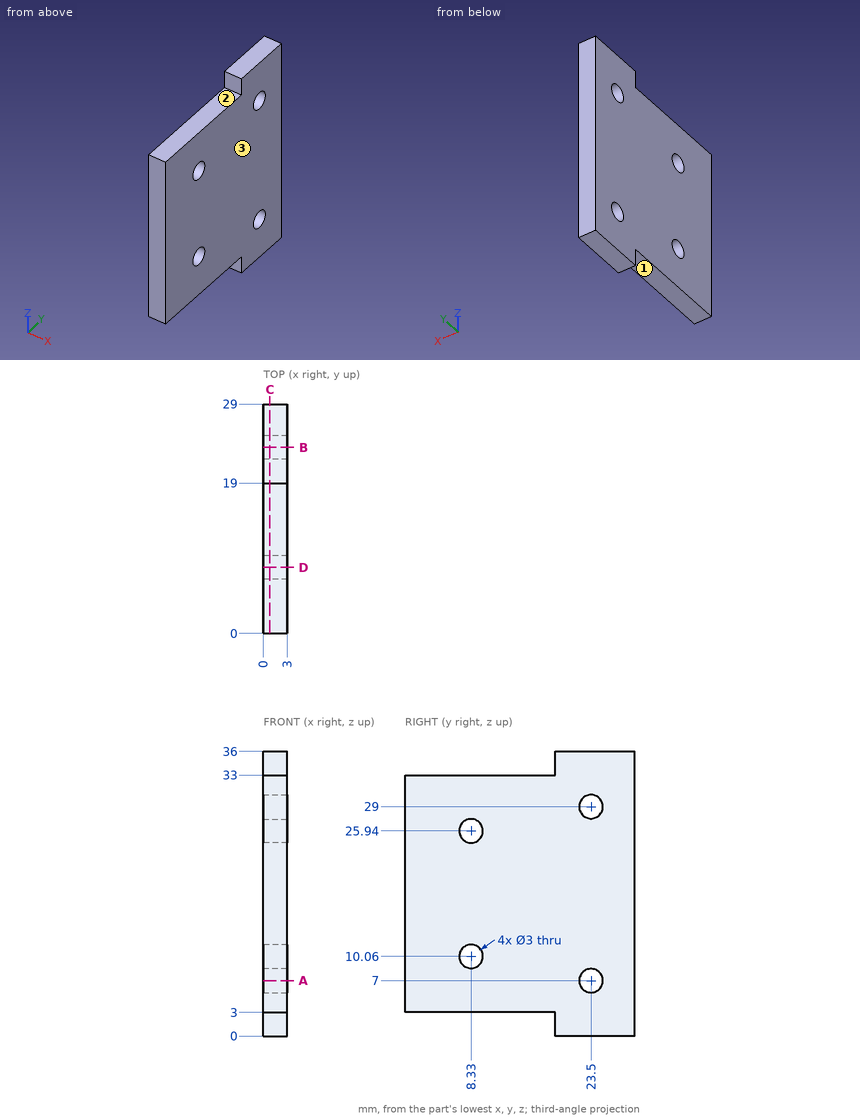
Source: three-view drawing plus pictorial views. Frame: mm from the lowest corner of the part. A direction names the side the tool comes from. Round coordinates to 2 decimals unless told otherwise and drop trailing zeros. Loops run counter-clockwise (first coordinate to the right, second up) from the corner with the lowest first, then second, coordinate; pieces in that order, holes last.
Q1. Section A-A on z = 7. Return loops of the section in (x, y), plus the area to 3 significant figures.
Q2. Section C-C on x = 0.8. Return loops of the section in (y, z).
Q3. Material intervals for L1, parallel to Y at x = 2.45, z = 29; L2, parallel to Z at x = 1.95, y = 7.5; L3, parallel to Y at x = 0.8, z = 10.06, sorted ascending.
Q4. Access query for the marked faces 1, 2 and 3. Directions: +Z, -Z, +X, -X, +Y, -Y. A direction counts if a zero-diameter tool reaches every point of the face in a straight line with its end or side. Return the directions, or none.
Q5. Pin query (flat end, axial travel): P1, Ø1.5, axis at x = 1.5, z = 34, coming from the -Y side; P2, Ø0.9, axis at x = 1.5, y = 10.5, coming from the +Z side. Return the tip coordinate at first contact, or that it passes through.
Q6. Section B-B on y = 23.5. Return loops of the section in (x, z).
Q7. Section D-D on y = 8.33. Return loops of the section in (x, z).
Evaluation:
1. outline: (0, 0) - (3, 0) - (3, 22) - (0, 22) - close; (0, 25) - (3, 25) - (3, 29) - (0, 29) - close
1. area: 78.0 mm2
2. outline: (0, 3) - (19, 3) - (19, 0) - (29, 0) - (29, 36) - (19, 36) - (19, 33) - (0, 33) - close; hole circle Ø3 at (8.33, 10.06); hole circle Ø3 at (8.33, 25.94); hole circle Ø3 at (23.5, 7); hole circle Ø3 at (23.5, 29)
3. L1: y = 0 to 22, 25 to 29
3. L2: z = 3 to 8.81, 11.31 to 24.69, 27.19 to 33
3. L3: y = 0 to 6.83, 9.83 to 29
4. face 1: -Z, +X, -X, -Y
4. face 2: +Z, +X, -X, -Y
4. face 3: +Z, -Z, +X, +Y, -Y
5. P1: stops at y = 19
5. P2: stops at z = 33
6. outline: (0, 0) - (3, 0) - (3, 5.5) - (0, 5.5) - close; (0, 8.5) - (3, 8.5) - (3, 27.5) - (0, 27.5) - close; (0, 30.5) - (3, 30.5) - (3, 36) - (0, 36) - close
7. outline: (0, 3) - (3, 3) - (3, 8.56) - (0, 8.56) - close; (0, 11.56) - (3, 11.56) - (3, 24.44) - (0, 24.44) - close; (0, 27.44) - (3, 27.44) - (3, 33) - (0, 33) - close
